Can you work these out from the drawing? Everything is in mm from the part's minimum corner. A direction names the side the tool comes from. Coordinates: 2 decimals unless noted, no trailing zeros. Loops run counter-clockwise (first coordinate to the right, second up) from the corner with the lowest first, then second, coordinate; pieces in that order, holes last.
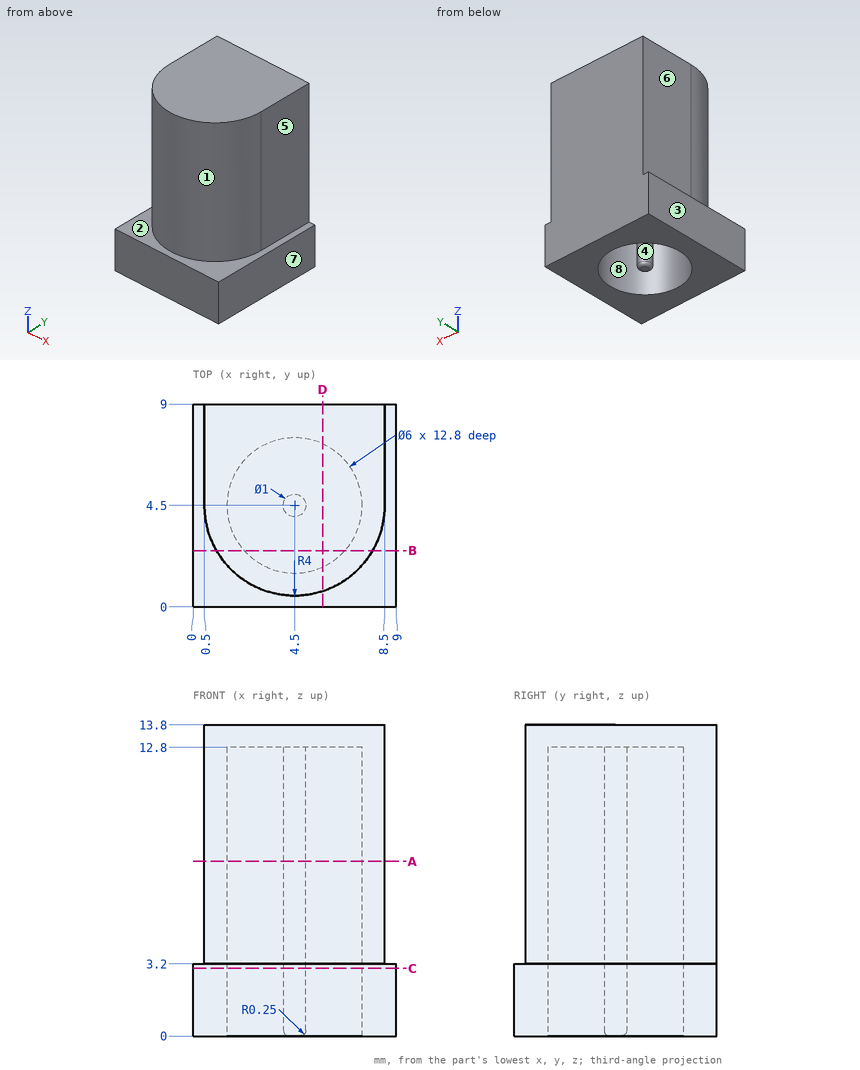
Item 1: We'd pull the mould along X, two halves only. Please class the marked faces 1, 2, 3 and 4: +X half, -X half, draft (parallel to the pull), parting line (faces both ways), or undercut.
Results are:
face 1: parting line
face 2: draft
face 3: -X half
face 4: undercut
Item 2: I'm going to push flat-ended pins straight in: P1, Ø1.5, axis at y = 4, z = 7, coming from the -X side; P2, Ø5, axis at y = 7, z = 7.5, coming from the +X side. Where does each tip first touch, or does it pass through?
Results are:
P1: stops at x = 0.5
P2: stops at x = 8.5
Item 3: Suppose I cut it at B-B, the plane y = 2.5. Please give me the cut outline in (x, z), plus the area to 3 significant figures.
Results are:
outline: (0, 0) - (2.26, 0) - (2.26, 12.8) - (6.74, 12.8) - (6.74, 0) - (9, 0) - (9, 3.2) - (7.96, 3.2) - (7.96, 13.8) - (1.04, 13.8) - (1.04, 3.2) - (0, 3.2) - close
area: 45.0 mm2
Item 4: I need wall thicknesses on line 1 along Y through (x, z) = (4.5, 9); line 2 along Y through (x, z) = (4.5, 3); line 3 along X through (y, z) = (7.75, 4.5). Which ranges of each line are inside material? Lowest first, please.
Results are:
line 1: y = 0.5 to 1.5, 4 to 5, 7.5 to 9
line 2: y = 0 to 1.5, 4 to 5, 7.5 to 9
line 3: x = 0.5 to 8.5
Item 5: On a 3-axis mill with a long thin cutter (end or side, diameter ignored), from which of +Z, -Z, +X, -X, +Y, -Y can I reach the whole of each face in a straight line? I mean the marked faces 5, 6, 7 and 8. Say none if no direction works.
Results are:
face 5: +Z, +X, +Y, -Y
face 6: +Z, -X, +Y, -Y
face 7: +Z, -Z, +X, +Y, -Y
face 8: -Z
Item 6: Suppose I cut it at A-A, the plane z = 7.75. Please give me the cut outline in (x, y).
Results are:
outline: (0.5, 4.5) arc R4 ccw to (8.5, 4.5) - (8.5, 9) - (0.5, 9) - close; circle Ø1 at (4.5, 4.5); hole circle Ø6 at (4.5, 4.5)
Item 7: Suppose I cut it at D-D, the plane x = 5.75. Please give me the cut outline in (y, z).
Results are:
outline: (0, 0) - (1.77, 0) - (1.77, 12.8) - (7.23, 12.8) - (7.23, 0) - (9, 0) - (9, 13.8) - (0.7, 13.8) - (0.7, 3.2) - (0, 3.2) - close
Item 8: Suppose I cut it at C-C, the plane z = 3. Please give me the cut outline in (x, y).
Results are:
outline: (0, 0) - (9, 0) - (9, 9) - (0, 9) - close; circle Ø1 at (4.5, 4.5); hole circle Ø6 at (4.5, 4.5)
